Check sheet for the drawn part. Datum: minimum x, y, z corner. Units: mm. A direction names the side the tool comes from. Give positions to 0.01 mm unless a question says otherwise; leave off trailing zeros. Loops run counter-clockwise (first coordinate to the right, second up) from the corner with the lowest first, then second, coordinate; pieces in that order, holes last. Notation, with made-up numbers: (86, -8.5) -> (142, -8.5) arc R10 cw to (142, 0.5) -> close; hole circle Ø1 at (76.5, 3.25). An arc over 180 degrees is marked (long way). One line per question, with ' | ' between items.
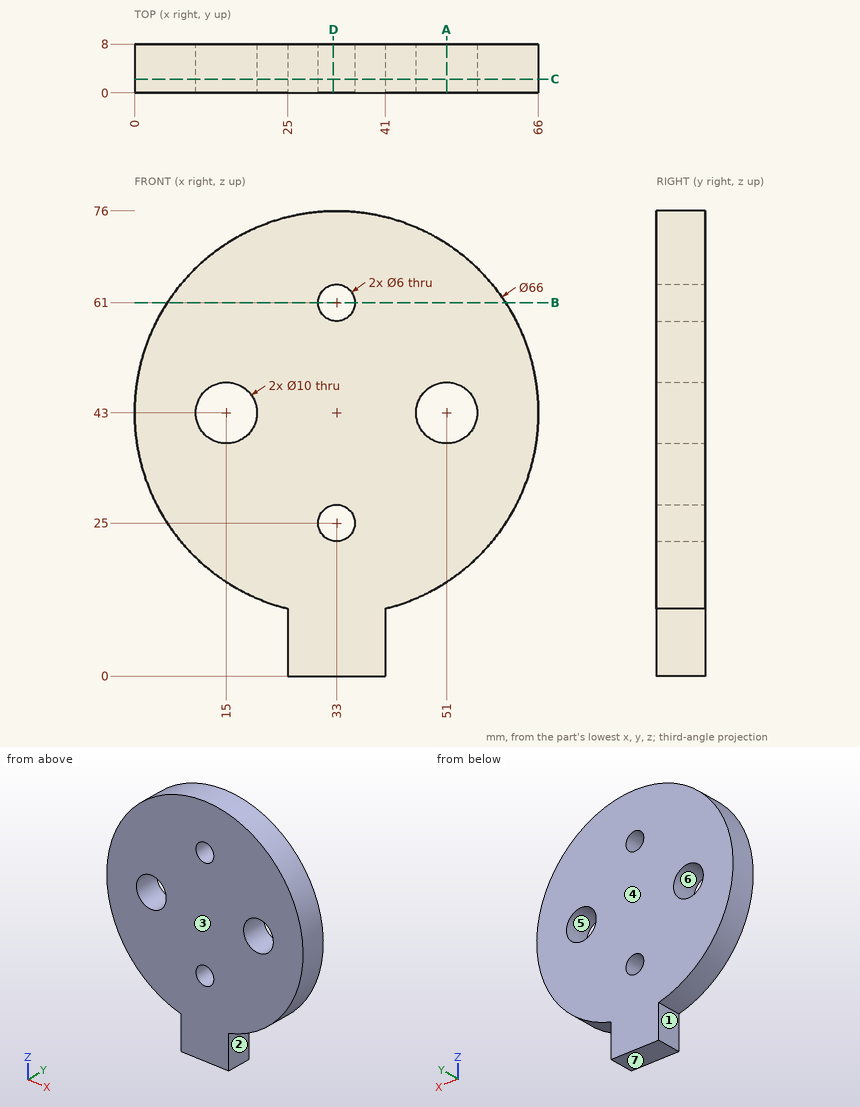
Item 1: Depth check by flat-ended pin: pin 1 Ø2.5 at (y, z) = (4.5, 8) entering from -X; pin 2 Ø4 at (y, z) = (2, 60.5) entering from -X; pin 3 Ø9 at (x, z) = (51, 43) entering from -Y; pin 4 Ø1 at (y, z) = (4, 63) entering from -X. Enter the tip coordinate at first touch or a pass-through.
Result:
pin 1: x = 25 | pin 2: x = 3.87 | pin 3: through | pin 4: x = 6.38
Item 2: Sectioned sample at D-D (x = 32.5). Record the cut outline in (y, z), plus the area to 3 significant figures.
Result:
outline: (0, 0) -> (8, 0) -> (8, 22.04) -> (0, 22.04) -> close; (0, 27.96) -> (8, 27.96) -> (8, 58.04) -> (0, 58.04) -> close; (0, 63.96) -> (8, 63.96) -> (8, 76) -> (0, 76) -> close | area: 513 mm2
Item 3: Set-up check for the marked faces 1, 2 and 3: record each of +Z, -Z, +X, -X, +Y, -Y from which the full face is reachable in a straight line by a thin tool's end or side.
Result:
face 1: -Z, -X, +Y, -Y | face 2: -Z, +X, +Y, -Y | face 3: +Z, -Z, +X, -X, -Y
Item 4: Scan lines: probe 1 along Z at (x, y) = (33, 2.5); probe 2 along X at (y, z) = (5.5, 43); probe 3 along X at (y, z) = (5, 46). Record each from-to range of solid material in increasing order.
Result:
probe 1: 0 to 22, 28 to 58, 64 to 76 | probe 2: 0 to 10, 20 to 46, 56 to 66 | probe 3: 0.14 to 11, 19 to 47, 55 to 65.86
Item 5: Sectioned sample at C-C (y = 2.25). Record the cut outline in (x, z), plus the area to 3 significant figures.
Result:
outline: (25, 0) -> (41, 0) -> (41, 10.98) arc R33 ccw (long way) to (25, 10.98) -> close; hole circle Ø10 at (15, 43); hole circle Ø6 at (33, 25); hole circle Ø6 at (33, 61); hole circle Ø10 at (51, 43) | area: 3,370 mm2
Item 6: Sectioned sample at A-A (x = 51). Record the cut outline in (y, z).
Result:
outline: (0, 15.34) -> (8, 15.34) -> (8, 38) -> (0, 38) -> close; (0, 48) -> (8, 48) -> (8, 70.66) -> (0, 70.66) -> close
Item 7: Sectioned sample at B-B (z = 61). Record the cut outline in (x, y), plus the area to 3 significant figures.
Result:
outline: (5.34, 0) -> (30, 0) -> (30, 8) -> (5.34, 8) -> close; (36, 0) -> (60.66, 0) -> (60.66, 8) -> (36, 8) -> close | area: 395 mm2
Item 8: Release check for a two-part mould opening along Z. For the marked faces 4, 5, 6 and 7 record: pulls with the +Z half, pulls with the -Z half, needs draft (parallel to the pull), parting line crosses it, or undercut.
Result:
face 4: needs draft | face 5: undercut | face 6: undercut | face 7: pulls with the -Z half
